from build123d import *

# Parameters (mm, degrees)
BOSS_EXTRUDE1_DEPTH = 6.35
CUT_EXTRUDE1_REACH  = 51.523
SKETCH2_R           = 16.0655
CUT_EXTRUDE2_REACH  = 51.523
SKETCH3_R           = 2.665
CUT_EXTRUDE3_REACH  = 51.523
SKETCH4_R           = 2.665
FILLET1_R           = 2.54


with BuildPart() as part:
    # Sketch1 → Boss-Extrude1 (new body)
    with BuildSketch(Plane(origin=(0, 0, 0), x_dir=(1, 0, 0), z_dir=(0, 1, 0))):
        with BuildLine():
            Line((-12.926329719, 25.4), (-40, 25.4))
            Line((-40, 25.4), (-40, -25.4))
            Line((-40, -25.4), (-12.926329719, -25.4))
            ThreePointArc((-12.926329719, -25.4), (0, -28.5), (12.926329719, -25.4))
            Line((12.926329719, -25.4), (40, -25.4))
            Line((40, -25.4), (40, 25.4))
            Line((40, 25.4), (12.926329719, 25.4))
            ThreePointArc((12.926329719, 25.4), (0, 28.5), (-12.926329719, 25.4))
        make_face()
    extrude(amount=BOSS_EXTRUDE1_DEPTH)

    # Sketch2 → Cut-Extrude1 (cut, up to next)
    with BuildSketch(Plane(origin=(0, 6.35, 0), x_dir=(1, 0, 0), z_dir=(0, 1, 0)), mode=Mode.PRIVATE) as cut_extrude1_sk1:
        with Locations(Location((0, 0, 0), (0, 0, 270))):
            Circle(SKETCH2_R)
    cut_extrude1_tool1 = extrude(cut_extrude1_sk1.sketch, amount=-CUT_EXTRUDE1_REACH, mode=Mode.PRIVATE) & part.part
    add(cut_extrude1_tool1.solids().sort_by_distance((0, 6.35, 0))[0], mode=Mode.SUBTRACT)

    # Sketch3 → Cut-Extrude2 (cut, up to next)
    with BuildSketch(Plane(origin=(0, 6.35, 0), x_dir=(1, 0, 0), z_dir=(0, 1, 0)), mode=Mode.PRIVATE) as cut_extrude2_sk1:
        with Locations(Location((0, 22.5, 0), (0, 0, 270))):
            Circle(SKETCH3_R)
    cut_extrude2_tool1 = extrude(cut_extrude2_sk1.sketch, amount=-CUT_EXTRUDE2_REACH, mode=Mode.PRIVATE) & part.part
    # Sketch3 → Cut-Extrude2 (cut, up to next)
    with BuildSketch(Plane(origin=(0, 6.35, 0), x_dir=(1, 0, 0), z_dir=(0, 1, 0)), mode=Mode.PRIVATE) as cut_extrude2_sk2:
        with Locations(Location((22.5, 0, 0), (0, 0, 270))):
            Circle(SKETCH3_R)
    cut_extrude2_tool2 = extrude(cut_extrude2_sk2.sketch, amount=-CUT_EXTRUDE2_REACH, mode=Mode.PRIVATE) & part.part
    # Sketch3 → Cut-Extrude2 (cut, up to next)
    with BuildSketch(Plane(origin=(0, 6.35, 0), x_dir=(1, 0, 0), z_dir=(0, 1, 0)), mode=Mode.PRIVATE) as cut_extrude2_sk3:
        with Locations(Location((0, -22.5, 0), (0, 0, 270))):
            Circle(SKETCH3_R)
    cut_extrude2_tool3 = extrude(cut_extrude2_sk3.sketch, amount=-CUT_EXTRUDE2_REACH, mode=Mode.PRIVATE) & part.part
    # Sketch3 → Cut-Extrude2 (cut, up to next)
    with BuildSketch(Plane(origin=(0, 6.35, 0), x_dir=(1, 0, 0), z_dir=(0, 1, 0)), mode=Mode.PRIVATE) as cut_extrude2_sk4:
        with Locations(Location((-22.5, 0, 0), (0, 0, 270))):
            Circle(SKETCH3_R)
    cut_extrude2_tool4 = extrude(cut_extrude2_sk4.sketch, amount=-CUT_EXTRUDE2_REACH, mode=Mode.PRIVATE) & part.part
    add(cut_extrude2_tool1.solids().sort_by_distance((0, 6.35, -22.5))[0], mode=Mode.SUBTRACT)
    add(cut_extrude2_tool2.solids().sort_by_distance((22.5, 6.35, 0))[0], mode=Mode.SUBTRACT)
    add(cut_extrude2_tool3.solids().sort_by_distance((0, 6.35, 22.5))[0], mode=Mode.SUBTRACT)
    add(cut_extrude2_tool4.solids().sort_by_distance((-22.5, 6.35, 0))[0], mode=Mode.SUBTRACT)

    # Sketch4 → Cut-Extrude3 (cut, up to next)
    with BuildSketch(Plane(origin=(0, 6.35, 0), x_dir=(1, 0, 0), z_dir=(0, 1, 0)), mode=Mode.PRIVATE) as cut_extrude3_sk1:
        with Locations(Location((-33.65, 19.05, 0), (0, 0, 270))):
            Circle(SKETCH4_R)
    cut_extrude3_tool1 = extrude(cut_extrude3_sk1.sketch, amount=-CUT_EXTRUDE3_REACH, mode=Mode.PRIVATE) & part.part
    # Sketch4 → Cut-Extrude3 (cut, up to next)
    with BuildSketch(Plane(origin=(0, 6.35, 0), x_dir=(1, 0, 0), z_dir=(0, 1, 0)), mode=Mode.PRIVATE) as cut_extrude3_sk2:
        with Locations(Location((-33.65, -19.05, 0), (0, 0, 270))):
            Circle(SKETCH4_R)
    cut_extrude3_tool2 = extrude(cut_extrude3_sk2.sketch, amount=-CUT_EXTRUDE3_REACH, mode=Mode.PRIVATE) & part.part
    # Sketch4 → Cut-Extrude3 (cut, up to next)
    with BuildSketch(Plane(origin=(0, 6.35, 0), x_dir=(1, 0, 0), z_dir=(0, 1, 0)), mode=Mode.PRIVATE) as cut_extrude3_sk3:
        with Locations(Location((33.65, 19.05, 0), (0, 0, 270))):
            Circle(SKETCH4_R)
    cut_extrude3_tool3 = extrude(cut_extrude3_sk3.sketch, amount=-CUT_EXTRUDE3_REACH, mode=Mode.PRIVATE) & part.part
    # Sketch4 → Cut-Extrude3 (cut, up to next)
    with BuildSketch(Plane(origin=(0, 6.35, 0), x_dir=(1, 0, 0), z_dir=(0, 1, 0)), mode=Mode.PRIVATE) as cut_extrude3_sk4:
        with Locations(Location((33.65, -19.05, 0), (0, 0, 270))):
            Circle(SKETCH4_R)
    cut_extrude3_tool4 = extrude(cut_extrude3_sk4.sketch, amount=-CUT_EXTRUDE3_REACH, mode=Mode.PRIVATE) & part.part
    add(cut_extrude3_tool1.solids().sort_by_distance((-33.65, 6.35, -19.05))[0], mode=Mode.SUBTRACT)
    add(cut_extrude3_tool2.solids().sort_by_distance((-33.65, 6.35, 19.05))[0], mode=Mode.SUBTRACT)
    add(cut_extrude3_tool3.solids().sort_by_distance((33.65, 6.35, -19.05))[0], mode=Mode.SUBTRACT)
    add(cut_extrude3_tool4.solids().sort_by_distance((33.65, 6.35, 19.05))[0], mode=Mode.SUBTRACT)

    # Fillet1
    fillet1_edges = [part.edges().sort_by_distance(p)[0] for p in [
        (12.926329719, 3.175, -25.4),
        (40, 3.175, -25.4),
        (40, 3.175, 25.4),
        (12.926329719, 3.175, 25.4),
        (-12.926329719, 3.175, 25.4),
        (-40, 3.175, 25.4),
        (-40, 3.175, -25.4),
        (-12.926329719, 3.175, -25.4),
    ]]
    fillet(fillet1_edges, radius=FILLET1_R)


solid = part.part
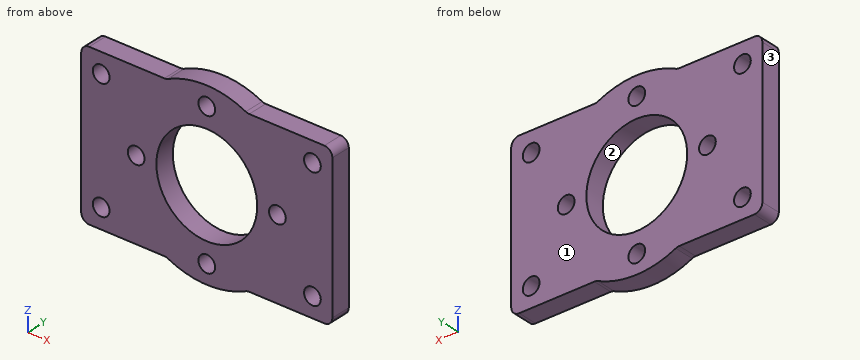
Design review of the part built by this model. Coordinates are the model's own, in mm. Face numbers are marked on the shaded views. Round coordinates to 2 decimals unless told otherwise and drop trailing zeros. Write each loop counter-clockwise with the first axis right and the second up, starting at its lowest first coordinate (ties: lowest second). Pieces come first, ordered by that corner, then holes. Notation, with made-up numbers: (61, -6) -> (94, -6) arc R27 ccw to (94, 33) -> close; hole circle Ø8 at (-13.75, -26.75). An arc over 180 degrees is marked (long way). One line per item, written item: value. Start each with the question number.
Q1. Insertion check: P1, Ø3, axis at x = 29, y = 4, coming from the +Z side. The pin has a flat end and moves straight along its axis. Give the tip position at first contact, or say it passes through.
Q2. Add section A-A (x = 0). State how many separate pieces and enclosed holes the cut face has, then the cut area to 3 significant figures.
Q3. To check wall thickness, follow probe 1 along X at (y, z) = (2, 0) (1 decimal); probe 2 along X at (y, z) = (2.75, -19.05) (3 decimals); probe 3 along X at (y, z) = (5.25, 22.5) (3 decimals). State the ranges of each line that lie inside material, in increasing order.
Q4. Add section D-D (x = -22.5). Give the boundary of the cut face in (y, z) (3 decimals), then the cut area to 3 significant figures.
Q5. The part is to be moulded in two halves that separate along X. For the marked faces 1, 2 and 3, say which applies: pulls with the +X half, pulls with the -X half, needs draft (parallel to the pull), parting line crosses it, or undercut.
Response:
1. P1: stops at z = 25.4
2. separate pieces: 4
2. enclosed holes: 0
2. area: 90.2 mm^2
3. probe 1: x = -40 to -25.2, -19.8 to -16.1, 16.1 to 19.8, 25.2 to 40
3. probe 2: x = -40 to -36.315, -30.985 to 30.985, 36.315 to 40
3. probe 3: x = -40 to -2.665, 2.665 to 40
4. outline: (0, -25.4) -> (6.35, -25.4) -> (6.35, -2.665) -> (0, -2.665) -> close; (0, 2.665) -> (6.35, 2.665) -> (6.35, 25.4) -> (0, 25.4) -> close
4. area: 289 mm^2
5. face 1: needs draft
5. face 2: undercut
5. face 3: pulls with the -X half
